Part model, mm, in its own coordinate system. A direction names the side the tool comes from. Coordinates: 2 decimals unless noted, no trailing zeros. Loops run counter-clockwise (first coordinate to the right, second up) from the corner with the lowest first, then second, coordinate; pieces in that order, holes last. Notation, with made-up numbers: M -8,81 L 13,81 A18 cw 13,111 Z; hole C -5.5,0.25 d9. An arc over 180 degrees is marked long. Use CSV: the item, a comma, the result in double quotes. Start each with the question number.
from build123d import *

# Parameters (mm, degrees)
SKETCH1_W                                    = 144
SKETCH1_H                                    = 270
BOSS_EXTRUDE1_DEPTH                          = 10
CBORE_FOR_M4_HEX_SOCKET_HEAD_CAP_SCR_2_COUNT = 2
CBORE_FOR_M4_HEX_SOCKET_HEAD_CAP_SCR_2_PITCH = 142.214626533
CBORE_FOR_M4_HEX_SOCKET_HEAD_CAP_SCR_3_COUNT = 2
CBORE_FOR_M4_HEX_SOCKET_HEAD_CAP_SCR_3_PITCH = 254
CBORE_FOR_M4_HEX_SOCKET_HEAD_CAP_SCR_4_COUNT = 2
CBORE_FOR_M4_HEX_SOCKET_HEAD_CAP_SCR_4_PITCH = 142.214626533
CUT_EXTRUDE1_REACH                           = 160.326
CUT_EXTRUDE1_START                           = -5
FILLET1_R                                    = 3


with BuildPart() as part:
    # Sketch1 → Boss-Extrude1 (new body)
    with BuildSketch(Plane.XY):
        Rectangle(SKETCH1_W, SKETCH1_H)
    extrude(amount=BOSS_EXTRUDE1_DEPTH)

    # Sketch3 → CBORE for M4 Hex Socket Head Cap Screw1 (revolve, cut)
    with BuildSketch(Plane(origin=(0, 127, 10), x_dir=(0, -1, 0), z_dir=(1, 0, 0))):
        Polygon((0, 0), (0, 10), (2.275, 10), (2.25, 9.975), (2.25, 4.4), (4, 4.4), (4, 0), align=None)
    cbore_for_m4_hex_socket_head_cap_screw1 = revolve(axis=Axis((0, 127, 16.35), (0, 0, -1)), mode=Mode.SUBTRACT)

    # CBORE for M4 Hex Socket Head Cap Scr 2: CBORE for M4 Hex Socket Head Cap Screw1 ×2
    with Locations(*[Vector(-0.4500240345181632, -0.8930164434969801, 0) * (i * CBORE_FOR_M4_HEX_SOCKET_HEAD_CAP_SCR_2_PITCH) for i in range(1, CBORE_FOR_M4_HEX_SOCKET_HEAD_CAP_SCR_2_COUNT)]):
        add(cbore_for_m4_hex_socket_head_cap_screw1, mode=Mode.SUBTRACT)

    # CBORE for M4 Hex Socket Head Cap Scr 3: CBORE for M4 Hex Socket Head Cap Screw1 ×2
    with Locations(*[(0, -i * CBORE_FOR_M4_HEX_SOCKET_HEAD_CAP_SCR_3_PITCH, 0) for i in range(1, CBORE_FOR_M4_HEX_SOCKET_HEAD_CAP_SCR_3_COUNT)]):
        add(cbore_for_m4_hex_socket_head_cap_screw1, mode=Mode.SUBTRACT)

    # CBORE for M4 Hex Socket Head Cap Scr 4: CBORE for M4 Hex Socket Head Cap Screw1 ×2
    with Locations(*[Vector(0.4500240345181632, -0.8930164434969801, 0) * (i * CBORE_FOR_M4_HEX_SOCKET_HEAD_CAP_SCR_4_PITCH) for i in range(1, CBORE_FOR_M4_HEX_SOCKET_HEAD_CAP_SCR_4_COUNT)]):
        add(cbore_for_m4_hex_socket_head_cap_screw1, mode=Mode.SUBTRACT)

    # Sketch4 → Cut-Extrude1 (cut, up to next)
    with BuildSketch(Plane.XY.offset(10).offset(CUT_EXTRUDE1_START), mode=Mode.PRIVATE) as cut_extrude1_sk1:
        with BuildLine():
            Line((-67, -6.32455532), (-67, -130))
            Line((-67, -130), (-6.32455532, -130))
            ThreePointArc((-6.32455532, -130), (0, -120), (6.32455532, -130))
            Line((6.32455532, -130), (67, -130))
            Line((67, -130), (67, -6.32455532))
            ThreePointArc((67, -6.32455532), (57, 0), (67, 6.32455532))
            Line((67, 6.32455532), (67, 130))
            Line((67, 130), (6.32455532, 130))
            ThreePointArc((6.32455532, 130), (0, 120), (-6.32455532, 130))
            Line((-6.32455532, 130), (-67, 130))
            Line((-67, 130), (-67, 6.32455532))
            ThreePointArc((-67, 6.32455532), (-57, 0), (-67, -6.32455532))
        make_face()
    cut_extrude1_tool1 = extrude(cut_extrude1_sk1.sketch, amount=-CUT_EXTRUDE1_REACH, mode=Mode.PRIVATE) & part.part
    add(cut_extrude1_tool1.solids().sort_by_distance((0, 0, 5))[0], mode=Mode.SUBTRACT)

    # Fillet1
    fillet1_edges = [part.edges().sort_by_distance(p)[0] for p in [
        (-72, 135, 5),
        (72, 135, 5),
        (72, -135, 5),
        (-72, -135, 5),
    ]]
    fillet(fillet1_edges, radius=FILLET1_R)


solid = part.part
1. Slice it at A-A, the plane z = 1.75. List the corners of the cut face in (x, y).
2. Wall check: probe 1 along X at (y, z) = (127, 4.05); probe 2 along X at (y, z) = (0, 1.85); probe 3 along Y at (x, z) = (0, 3.35). Give the ranges that are in metal, low to high.
3. Slice it at B-B, the plane y = -48. List the corners of the cut face in (x, z), and give its area (3 significant figures).
4. Tool access for faces 1 (the face through (-1, 135, 5)), 2 (the face through (36, -130, 3)), 3 (the face through (-62, 2, 5.6)): list every direction of +Z, -Z, +X, -X, +Y, -Y with a clear straight run to the whole face (end or side of a thin tool).
5. Pin check, flat tips, straight feed: pin 1 (7 mm diameter, centred on x = 0, y = 127, fed in from +Z); pin 2 (3.5 mm diameter, centred on x = 64, y = 0, fed in from +Z); pin 3 (12 mm diameter, centred on x = 30, y = -92.5, fed in from -Z). Stop position of each tip, or through.
6. Slice it at C-C, the plane x = -37. List the corners of the cut face in (y, z), and give its area (3 significant figures).
7. Two-plate mould, pull along X, no slides. Class faces 4 (the face through (-1, 2, 10)), 5 (the face through (0, 120, 3)): pulls with the +X half, pulls with the -X half, needs draft (parallel to the pull), parting line crosses it, or undercut.
Found:
1,outline,"M -72,-132 A3 ccw -69,-135 L 69,-135 A3 ccw 72,-132 L 72,132 A3 ccw 69,135 L -69,135 A3 ccw -72,132 Z; hole M -67,-130 L -6.32,-130 A7 cw long 6.32,-130 L 67,-130 L 67,-6.32 A7 cw long 67,6.32 L 67,130 L 6.32,130 A7 cw long -6.32,130 L -67,130 L -67,6.32 A7 cw long -67,-6.32 Z; hole C -64,0 d4.5; hole C 0,-127 d4.5; hole C 0,127 d4.5; hole C 64,0 d4.5"
2,probe 1,"-72 to -67, -7 to -2.25, 2.25 to 7, 67 to 72"
2,probe 2,"-72 to -66.25, -61.75 to -57, 57 to 61.75, 66.25 to 72"
2,probe 3,"-135 to -129.25, -124.75 to -120, 120 to 124.75, 129.25 to 135"
3,outline,"M -72,0 L -67,0 L -67,5 L 67,5 L 67,0 L 72,0 L 72,10 L -72,10 Z"
3,area,"770 mm^2"
4,face 1,"+Z, -Z, +X, -X, +Y"
4,face 2,"-Z"
4,face 3,"+Z"
5,pin 1,"z = 5.6"
5,pin 2,"through"
5,pin 3,"z = 5"
6,outline,"M -135,0 L -130,0 L -130,5 L 130,5 L 130,0 L 135,0 L 135,10 L -135,10 Z"
6,area,"1,400 mm^2"
7,face 4,"needs draft"
7,face 5,"undercut"
